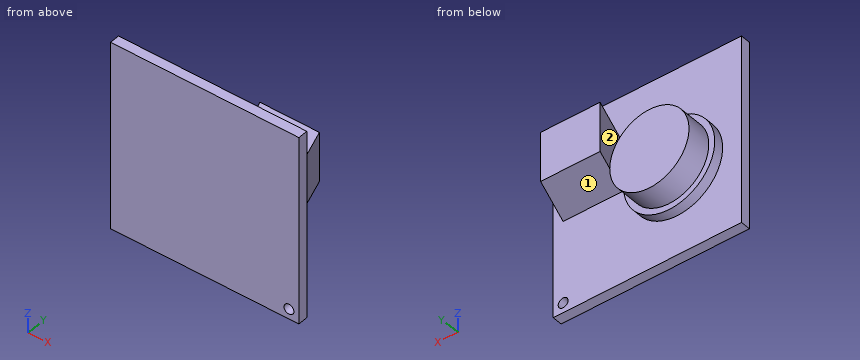
from build123d import *

# Parameters (mm, degrees)
SKETCH_1_W          = 19
SKETCH_1_H          = 19
EXTRUDE_1_DEPTH     = 1
SKETCH_2_R          = 0.5
CUT_EXTRUDE_1_DEPTH = 1
SKETCH_3_R          = 4.6
EXTRUDE_2_DEPTH     = 1
SKETCH_5_R          = 4
EXTRUDE_3_DEPTH     = 2.5
SKETCH_6_W          = 6
SKETCH_6_H          = 5


with BuildPart() as part:
    # Эскиз1 → Бобышка-Вытянуть1 (new body)
    with BuildSketch(Plane(origin=(0, 0, 0), x_dir=(1, 0, 0), z_dir=(0, 1, 0))):
        with Locations((-26.569127832, -17.007177836)):
            Rectangle(SKETCH_1_W, SKETCH_1_H)
    extrude(amount=EXTRUDE_1_DEPTH)

    # Эскиз2 → Вырез-Вытянуть1 (cut)
    with BuildSketch(Plane(origin=(0, 1, 0), x_dir=(1, 0, 0), z_dir=(0, 1, 0))):
        with Locations((-18.069127832, -8.507177836)):
            Circle(SKETCH_2_R)
    extrude(amount=-CUT_EXTRUDE_1_DEPTH, mode=Mode.SUBTRACT)

    # Эскиз3 → Бобышка-Вытянуть2 (add)
    with BuildSketch(Plane(origin=(0, 1, 0), x_dir=(1, 0, 0), z_dir=(0, 1, 0))):
        with Locations((-29.569127832, -16.107177836)):
            Circle(SKETCH_3_R)
    extrude(amount=EXTRUDE_2_DEPTH)

    # Эскиз5 → Бобышка-Вытянуть3 (add)
    with BuildSketch(Plane(origin=(0, 2, 0), x_dir=(1, 0, 0), z_dir=(0, 1, 0))):
        with Locations((-29.569127832, -16.107177836)):
            Circle(SKETCH_5_R)
    extrude(amount=EXTRUDE_3_DEPTH)

    # По траектории1: sweep along a path in Эскиз9
    with BuildLine(Plane.XY) as sweep_1_path:
        Line((-24.069127832, 1), (-25.789600147, 6))
    # Эскиз6 → По траектории1 (sweep)
    with BuildSketch(Plane(origin=(0, 1, 0), x_dir=(1, 0, 0), z_dir=(0, 1, 0))):
        with Locations((-21.069127832, -19.307177836)):
            Rectangle(SKETCH_6_W, SKETCH_6_H)
    sweep(path=sweep_1_path.line)


solid = part.part
Check sheet for the modelled part. Datum: model origin and axes. Units: mm. Face numbers are marked on the shaded views. Round coordinates to 2 decimals unless told otherwise and drop trailing zeros. Loops run counter-clockwise (first coordinate to the right, second up) from the corner with the lowest first, then second, coordinate; pieces in that order, holes last. Notation, with made-up numbers: M 57,68.25 L 86,68.25 A13 ccw 86,74.25 Z; hole C 83.25,18 d9. An arc over 180 degrees is marked long. One line per question, with ' | ' between items. Start each with the question number.
Item 1: Section check C-C (z = 19). Record the boundary of the cut face in (x, y), and give its area (3 significant figures).
Item 2: Scan lines: probe 1 along Y at (x, z) = (-26.5, 23.5); probe 2 along Z at (x, y) = (-19.75, 3.15); probe 3 along X at (y, z) = (1.6, 18.75). Record each from-to range of solid material in increasing order.
Item 3: Section check D-D (x = -27.75). Record the boundary of the cut face in (y, z).
Item 4: Gauge pin test, flat ends, axial feed: pin 1 Ø2.5 at (x, y) = (-23, 4.5) entering from -Z; pin 2 Ø7.5 at (x, z) = (-29.5, 16) entering from +Y; pin 3 Ø1 at (y, z) = (3, 10) entering from -X; pin 4 Ø5.5 at (x, z) = (-23.5, 12.5) entering from +Y. Record the tip position at first contact, or that the pin passes through.
Item 5: Release check for a two-part mould opening along X. For the marked faces 1 and 2 record: released by +X, released by -X, zero draft, split by the parting line, or undercut.
Item 6: Section check A-A (x = -30.75). Record the boundary of the cut face in (y, z), and give its area (3 significant figures).
Item 7: Section check B-B (y = 2.95). Record the boundary of the cut face in (x, z).
Worked out:
1) outline: M -36.07,0 L -17.07,0 L -17.07,1 L -18.07,1 L -19.79,6 L -25.79,6 L -24.07,1 L -25.99,1 L -25.99,2 L -26.81,2 L -26.81,4.5 L -32.33,4.5 L -32.33,2 L -33.15,2 L -33.15,1 L -36.07,1 Z | area: 70.0 mm^2
2) probe 1: 0 to 1 | probe 2: 16.81 to 21.81 | probe 3: -33.33 to -25.8, -24.28 to -18.28
3) outline: M 0,7.51 L 1,7.51 L 1,11.88 L 2,11.88 L 2,12.54 L 4.5,12.54 L 4.5,19.67 L 2,19.67 L 2,20.33 L 1,20.33 L 1,26.51 L 0,26.51 Z
4) pin 1: z = 16.81 | pin 2: y = 4.5 | pin 3: through | pin 4: y = 2
5) face 1: zero draft | face 2: undercut
6) outline: M 0,7.51 L 1,7.51 L 1,11.66 L 2,11.66 L 2,12.29 L 4.5,12.29 L 4.5,19.93 L 2,19.93 L 2,20.55 L 1,20.55 L 1,26.51 L 0,26.51 Z | area: 47.0 mm^2
7) outline: C -29.57,16.11 d8; M -24.74,16.81 L -18.74,16.81 L -18.74,21.81 L -24.74,21.81 Z
